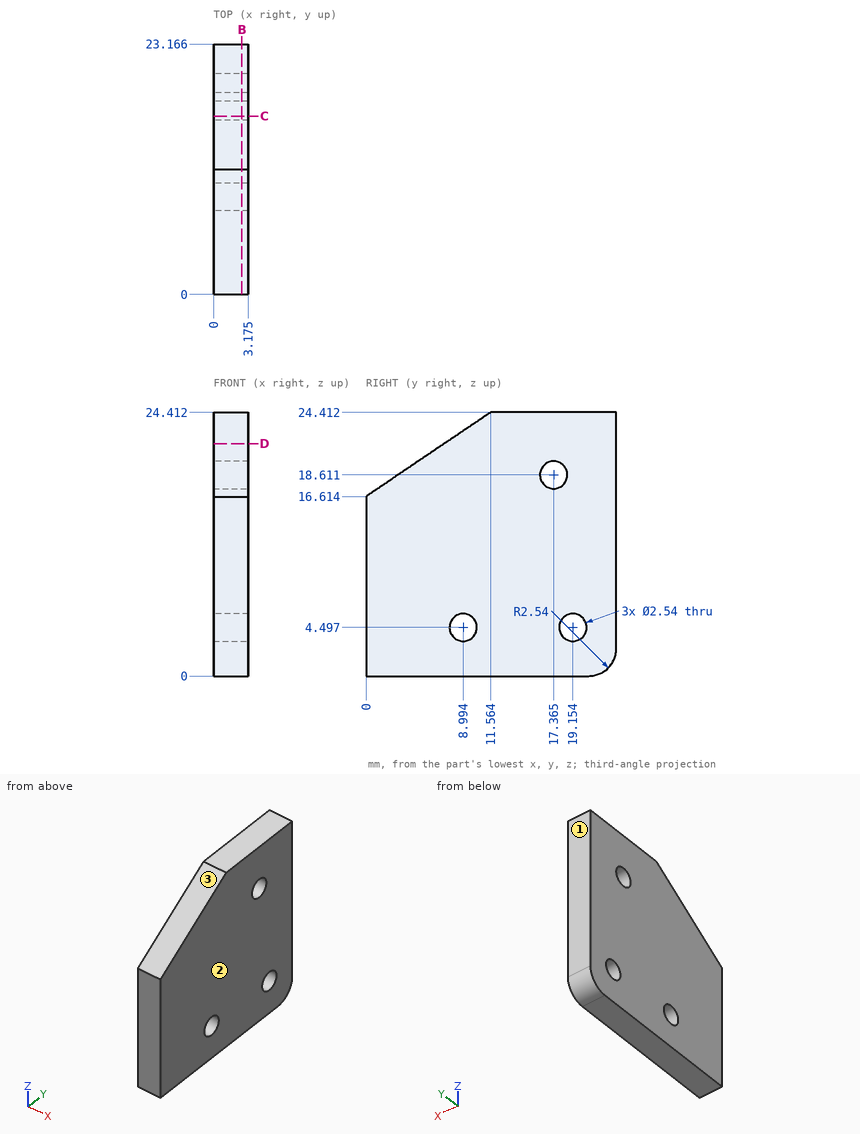
Check sheet for the drawn part. Datum: minimum x, y, z corner. Units: mm. Give positions to 0.01 mm unless a question says otherwise; leave off trailing zeros. Write each loop counter-clockwise with the first axis right and the second up, starting at its lowest first coordinate (ties: lowest second). Pieces come first, ordered by that corner, then holes.
(1) Gauge pin test, flat ends, axial feed: pin 1 (3 mm diameter, centred on y = 8.99, z = 4.5, fed in from -X); pin 2 (1.5 mm diameter, centred on x = 2, y = 6.5, fed in from +Z). Record the tip position at first contact, or that the pin passes through.
(2) Cross-section at B-B (x = 2.6). Enter the section's corners in (y, z) (1 decimal), plus the area to 3 significant figures.
(3) Cross-section at C-C (y = 16.5). Enter the section's corners in (x, z) (1 decimal).
(4) Material ranges on line 1 (Z direction, x = 2.45, y = 19.5) (1 decimal); line 2 (Y direction, x = 2.4, z = 19.5) (1 decimal); line 3 (Z direction, x = 1.3, y = 6), recorded low to high.
(5) Cross-section at D-D (z = 21.5). Enter the section's corners in (x, y) (1 decimal).
(6) Mould release check, pull along Y, two halves, no side actions. Record for the marked faces 1, 2 and 3: +Y half, -Y half, draft (parallel to the pull), parting line (faces both ways), or undercut.
Worked out:
1. pin 1: stops at x = 0
1. pin 2: stops at z = 21.5
2. outline: (0, 0) - (20.6, 0) arc R2.5 ccw to (23.2, 2.5) - (23.2, 24.4) - (11.6, 24.4) - (0, 16.6) - close; hole circle Ø2.5 at (9, 4.5); hole circle Ø2.5 at (17.4, 18.6); hole circle Ø2.5 at (19.2, 4.5)
2. area: 504 mm2
3. outline: (0, 0) - (3.2, 0) - (3.2, 17.7) - (0, 17.7) - close; (0, 19.5) - (3.2, 19.5) - (3.2, 24.4) - (0, 24.4) - close
4. line 1: z = 0 to 3.3, 5.7 to 24.4
4. line 2: y = 4.3 to 16.5, 18.3 to 23.2
4. line 3: z = 0 to 20.66
5. outline: (0, 7.2) - (3.2, 7.2) - (3.2, 23.2) - (0, 23.2) - close
6. face 1: +Y half
6. face 2: draft
6. face 3: -Y half
